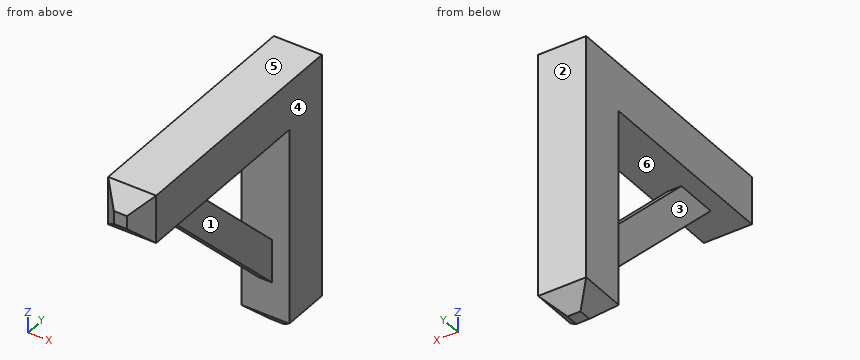
from build123d import *

# Parameters (mm, degrees)
F1_DEPTH = 69.85
F2_SIZE2 = 50.8
F2_SIZE  = 50.8
F4_DEPTH = 19.05
F5_SCALE = 0.0114810563


with BuildPart() as f1:
    # F0 (on Right) → F1 (new body, symmetric)
    with BuildSketch(Plane.YZ):
        Polygon((0, 0), (-762, 0), (-762, -139.7), (-139.7, -139.7), (-139.7, -762), (0, -762), align=None)
    extrude(amount=F1_DEPTH, both=True)

    # F2
    f2_edges = [f1.edges().sort_by_distance(p)[0] for p in [
        (0, -762, -139.7),
        (69.85, -69.85, -762),
        (0, -139.7, -762),
        (-69.85, -69.85, -762),
        (0, 0, -762),
        (-69.85, -762, -69.85),
        (0, -762, 0),
        (69.85, -762, -69.85),
    ]]
    chamfer(f2_edges, length=F2_SIZE, length2=F2_SIZE2)

    # F3 (on Right) → F4 (join, symmetric)
    with BuildSketch(Plane.YZ):
        Polygon((-483.876414305, -139.7), (-609.6, -139.7), (-139.7, -609.6), (-139.7, -483.876414305), align=None)
    extrude(amount=F4_DEPTH, both=True)


with BuildPart() as f1_1:
    # F5: moved
    add(f1.part.scale(F5_SCALE))


solid = f1_1.part
Design review of the part built by this model. Coordinates are the model's own, in mm. Face numbers are marked on the shaded views. A direction names the side the tool comes from. Round coordinates to 2 decimals unless told otherwise and drop trailing zeros. Loops run counter-clockwise (first coordinate to the right, second up) from the corner with the lowest first, then second, coordinate; pieces in that order, holes last. Notation, with made-up numbers: M 62,58 L 69,58 A17 ccw 69,71 Z; hole C 83,7 d3. An arc over 180 degrees is marked long. Answer as a JSON object with one key per item and string values.
Item 1: Wall thickness on L1, parallel to Y at x = -0.45, z = -8; L2, parallel to X at y = -4.5, z = -3.75; L3, parallel to Z at x = 0, y = -2.5: over which ranges is each line inside the solid? List them lowest first. Write a range as from..to.
Answer sheet:
{"L1": "y = -1.6..0", "L2": "x = -0.22..0.22", "L3": "z = -6.1..-4.66, -1.6..0"}
Item 2: The part is to be moulded in two halves that separate along Z. For the marked faces 4, 5 and 6, say which applies: pulls with the +Z half, pulls with the -Z half, needs draft (parallel to the pull), parting line crosses it, or undercut.
Answer sheet:
{"face 4": "needs draft", "face 5": "pulls with the +Z half", "face 6": "undercut"}
Item 3: Machinability: for the marked faces 1, 2 and 3, which of the approach directions +Z, -Z, +X, -X, +Y, -Y give a long, thin tool a straight path to every point of the face, cutting with its end or side? Answer none if there is none.
Answer sheet:
{"face 1": "-Z, +X, -Y", "face 2": "+Z, -Z, +X, -X, +Y", "face 3": "-Z, -X, -Y"}
Item 4: We need section A-A on z = -4.5. Give the boundary of the cut face in (x, y).
Answer sheet:
{"outline": "M -0.8,-1.6 L 0.8,-1.6 L 0.8,0 L -0.8,0 Z; M -0.22,-4.1 L 0.22,-4.1 L 0.22,-2.66 L -0.22,-2.66 Z"}
Item 5: We need section C-C on x = -0.6. Give the boundary of the cut face in (y, z), and give its area (3 significant figures).
Answer sheet:
{"outline": "M -8.37,-1.4 L -8.17,-1.6 L -1.6,-1.6 L -1.6,-8.17 L -1.4,-8.37 L -0.2,-8.37 L 0,-8.17 L 0,0 L -8.17,0 L -8.37,-0.2 Z", "area": "24.2 mm^2"}
Item 6: We need section B-B on y = -2. Give the boundary of the cut face in (x, z).
Answer sheet:
{"outline": "M -0.8,-1.6 L 0.8,-1.6 L 0.8,0 L -0.8,0 Z; M -0.22,-6.6 L 0.22,-6.6 L 0.22,-5.16 L -0.22,-5.16 Z"}
Item 7: We need section D-D on z = -6.5. Give the boundary of the cut face in (x, y).
Answer sheet:
{"outline": "M -0.8,-1.6 L -0.22,-1.6 L -0.22,-2.1 L 0.22,-2.1 L 0.22,-1.6 L 0.8,-1.6 L 0.8,0 L -0.8,0 Z"}
